```python
from build123d import *

# Parameters (mm, degrees)
SKETCH1_W               = 46.5
SKETCH1_H               = 24
BOSS_EXTRUDE1_DEPTH     = 21
SHELL1_T                = -1.25
SKETCH2_W               = 19.75
SKETCH2_H               = 14.5
CUT_EXTRUDE1_DEPTH      = 57.384838388
CUT_EXTRUDE4_REACH      = 57.358
SKETCH6_R               = 1.95
CUT_EXTRUDE5_REACH      = 57.358
SKETCH7_W               = 10.375
SKETCH7_H               = 2.5
SKETCH9_W               = 19.5
SKETCH9_H               = 6
BOSS_EXTRUDE3_DEPTH     = 2.5
CUT_EXTRUDE7_DEPTH      = 102.634838388
CUT_EXTRUDE7_DEPTH_BACK = 57.384838388
CUT_EXTRUDE7_START      = -45.25
SKETCH12_W              = 1.5
SKETCH12_H              = 8.25
SKETCH13_W              = 2.75
SKETCH13_H              = 8.25
BOSS_EXTRUDE4_DEPTH     = 44
SKETCH15_W              = 10
SKETCH15_H              = 2.75
BOSS_EXTRUDE5_DEPTH     = 0.75
CUT_EXTRUDE8_REACH      = 57.358
SKETCH18_W              = 6.76
SKETCH18_H              = 5
CUT_EXTRUDE9_REACH      = 57.358
SKETCH22_W              = 8.593751287
SKETCH22_H              = 16.011767213
CUT_EXTRUDE15_REACH     = 57.358
SKETCH25_W              = 10
SKETCH25_H              = 4.5


with BuildPart() as part:
    # Sketch1 → Boss-Extrude1 (new body)
    with BuildSketch(Plane.XY):
        with Locations((22, 12)):
            Rectangle(SKETCH1_W, SKETCH1_H)
    extrude(amount=-BOSS_EXTRUDE1_DEPTH)

    # Shell1
    shell1_openings = [part.faces().sort_by_distance(p)[0] for p in [
        (22, 12, -21),
        (22, 24, -10.5),
    ]]
    offset(amount=SHELL1_T, openings=shell1_openings, kind=Kind.INTERSECTION)

    # Sketch2 → Cut-Extrude1 (cut, through all)
    with BuildSketch(Plane.ZY.offset(1.25)):
        with Locations((-11.125, 8.5)):
            Rectangle(SKETCH2_W, SKETCH2_H)
    extrude(amount=-CUT_EXTRUDE1_DEPTH, mode=Mode.SUBTRACT)

    # Sketch6 → Cut-Extrude4 (cut, up to next)
    with BuildSketch(Plane(origin=(0, 0, 0), x_dir=(-1, 0, 0), z_dir=(0, -1, 0)), mode=Mode.PRIVATE) as cut_extrude4_sk1:
        with Locations(Location((-6.125, 9, 0), (0, 0, 90))):
            Circle(SKETCH6_R)
    cut_extrude4_tool1 = extrude(cut_extrude4_sk1.sketch, amount=-CUT_EXTRUDE4_REACH, mode=Mode.PRIVATE) & part.part
    # Sketch6 → Cut-Extrude4 (cut, up to next)
    with BuildSketch(Plane(origin=(0, 0, 0), x_dir=(-1, 0, 0), z_dir=(0, -1, 0)), mode=Mode.PRIVATE) as cut_extrude4_sk2:
        with Locations(Location((-37.875, 9, 0), (0, 0, 90))):
            Circle(SKETCH6_R)
    cut_extrude4_tool2 = extrude(cut_extrude4_sk2.sketch, amount=-CUT_EXTRUDE4_REACH, mode=Mode.PRIVATE) & part.part
    add(cut_extrude4_tool1.solids().sort_by_distance((6.125, 0, -9))[0], mode=Mode.SUBTRACT)
    add(cut_extrude4_tool2.solids().sort_by_distance((37.875, 0, -9))[0], mode=Mode.SUBTRACT)

    # Sketch7 → Cut-Extrude5 (cut, up to next)
    with BuildSketch(Plane.XY, mode=Mode.PRIVATE) as cut_extrude5_sk1:
        with Locations((40.0625, 2.5)):
            Rectangle(SKETCH7_W, SKETCH7_H)
    cut_extrude5_tool1 = extrude(cut_extrude5_sk1.sketch, amount=-CUT_EXTRUDE5_REACH, mode=Mode.PRIVATE) & part.part
    # Sketch7 → Cut-Extrude5 (cut, up to next)
    with BuildSketch(Plane.XY, mode=Mode.PRIVATE) as cut_extrude5_sk2:
        with Locations((3.9375, 2.5)):
            Rectangle(SKETCH7_W, SKETCH7_H)
    cut_extrude5_tool2 = extrude(cut_extrude5_sk2.sketch, amount=-CUT_EXTRUDE5_REACH, mode=Mode.PRIVATE) & part.part
    add(cut_extrude5_tool1.solids().sort_by_distance((40.0625, 2.5, 0))[0], mode=Mode.SUBTRACT)
    add(cut_extrude5_tool2.solids().sort_by_distance((3.9375, 2.5, 0))[0], mode=Mode.SUBTRACT)

    # Sketch9 → Boss-Extrude3 (add)
    with BuildSketch(Plane(origin=(0, 1.25, 0), x_dir=(1, 0, 0), z_dir=(0, 1, 0))):
        with Locations((25.125, 18)):
            Rectangle(SKETCH9_W, SKETCH9_H)
    extrude(amount=BOSS_EXTRUDE3_DEPTH)

    # Sketch12 → Cut-Extrude7 (cut, two sides: drawn at the far end of the back side and taken through both)
    with BuildSketch(Plane(origin=(45.25, 0, 0), x_dir=(0, 0, -1), z_dir=(1, 0, 0)).offset(CUT_EXTRUDE7_START - CUT_EXTRUDE7_DEPTH_BACK)):
        with Locations((20.25, 19.875)):
            Rectangle(SKETCH12_W, SKETCH12_H)
    extrude(amount=CUT_EXTRUDE7_DEPTH + CUT_EXTRUDE7_DEPTH_BACK, mode=Mode.SUBTRACT)

    # Sketch13 → Boss-Extrude4 (add)
    with BuildSketch(Plane(origin=(0, 0, 0), x_dir=(0, 0, -1), z_dir=(1, 0, 0))):
        with Locations((18.125, 19.875)):
            Rectangle(SKETCH13_W, SKETCH13_H)
    extrude(amount=BOSS_EXTRUDE4_DEPTH)

    # Sketch15 → Boss-Extrude5 (add)
    with BuildSketch(Plane.XZ.offset(-15.75)):
        with Locations((29.875, -18.125)):
            Rectangle(SKETCH15_W, SKETCH15_H)
    extrude(amount=BOSS_EXTRUDE5_DEPTH)

    # Sketch18 → Cut-Extrude8 (cut, up to next)
    with BuildSketch(Plane.XY, mode=Mode.PRIVATE) as cut_extrude8_sk1:
        with Locations((9.98, 10.1)):
            Rectangle(SKETCH18_W, SKETCH18_H)
    cut_extrude8_tool1 = extrude(cut_extrude8_sk1.sketch, amount=-CUT_EXTRUDE8_REACH, mode=Mode.PRIVATE) & part.part
    add(cut_extrude8_tool1.solids().sort_by_distance((9.98, 10.1, 0))[0], mode=Mode.SUBTRACT)

    # Sketch22 → Cut-Extrude9 (cut, up to next)
    with BuildSketch(Plane.XY, mode=Mode.PRIVATE) as cut_extrude9_sk1:
        with Locations((21.422492142, 15.994116394)):
            Rectangle(SKETCH22_W, SKETCH22_H)
    cut_extrude9_tool1 = extrude(cut_extrude9_sk1.sketch, amount=-CUT_EXTRUDE9_REACH, mode=Mode.PRIVATE) & part.part
    add(cut_extrude9_tool1.solids().sort_by_distance((21.422492, 15.994116, 0))[0], mode=Mode.SUBTRACT)

    # Sketch25 → Cut-Extrude15 (cut, up to next)
    with BuildSketch(Plane.XY, mode=Mode.PRIVATE) as cut_extrude15_sk1:
        Polygon((31.35, 18.75), (41.85, 18.75), (41.85, 24), (41.6, 24), (41.6, 19.5), (31.6, 19.5), (31.6, 24), (31.35, 24), align=None)
    cut_extrude15_tool1 = extrude(cut_extrude15_sk1.sketch, amount=-CUT_EXTRUDE15_REACH, mode=Mode.PRIVATE) & part.part
    # Sketch25 → Cut-Extrude15 (cut, up to next)
    with BuildSketch(Plane.XY, mode=Mode.PRIVATE) as cut_extrude15_sk2:
        with Locations((36.6, 21.75)):
            Rectangle(SKETCH25_W, SKETCH25_H)
    cut_extrude15_tool2 = extrude(cut_extrude15_sk2.sketch, amount=-CUT_EXTRUDE15_REACH, mode=Mode.PRIVATE) & part.part
    add(cut_extrude15_tool1.solids().sort_by_distance((31.475, 23.882606, 0))[0], mode=Mode.SUBTRACT)
    add(cut_extrude15_tool2.solids().sort_by_distance((36.6, 21.75, 0))[0], mode=Mode.SUBTRACT)


solid = part.part
```
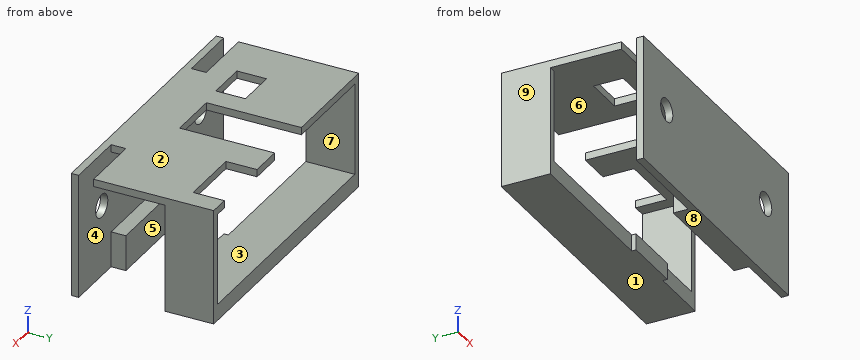
Geometry check sheet. Reference: the model listing, model coordinates, mm. Face numbers are marked on the shaded views. A direction names the side the tool comes from. Coordinates: 2 decimals unless noted, no trailing zeros. Loops run counter-clockwise (first coordinate to the right, second up) from the corner with the lowest first, then second, coordinate; pieces in that order, holes last. Notation, with made-up numbers: (-5.75, 11.25) - (37.25, 11.25) arc R28 ccw to (37.25, 30.25) - close; hole circle Ø6 at (59.25, 52.25). An arc over 180 degrees is marked (long way). One line per item, written item: value. Start each with the question number.
(1) Tool access check on the marked faces 1, 2, 3, 4 and 5. Record the directions out of +Z, -Z, +X, -X, +Y, -Y that give a thin tool (end or side, any length) a straight path to the whole face; none if there is none.
(2) Cross-section at B-B on y = 20. Enter the section's corners in (x, z).
(3) Mould release check, pull along Z, two halves, no side actions. Record for the marked faces 6, 7, 8 and 9: released by +Z, released by -Z, zero draft, split by the parting line, or undercut.
(4) Cross-section at A-A on z = -2.5. Enter the section's corners in (x, y), plus the area to 4 significant figures.
(5) Material ranges on line 1 (X direction, y = 0.9, z = -9) (3 decimals); line 2 (Y direction, x = 43.5, z = -17.25); line 3 (Y direction, x = 28, z = -19.25), recorded low to high. Write a range as [from, to].
(6) Cross-section at C-C on z = -9. Enter the section's corners in (x, y) (3 decimals).
(7) Cross-section at D-D on z = -17.5. Enter the section's corners in (x, y) (3 decimals), plus the area to 3 significant figures.
(8) Depth check by flat-ended pin: P1, Ø6, axis at x = 40.5, z = -16, coming from the -Y side; P2, Ø2, axis at x = 39.5, y = 12, coming from the -Z side; P3, Ø1.4, axis at y = 2.5, z = -0.5, coming from the -X side (3 decimals); P4, Ø2, axis at y = 14.5, z = -18, coming from the +X side (3 decimals). Enter the tip coordinate at first touch or a pass-through.
Results below:
1. face 1: -Z, +X, -X, +Y
1. face 2: +Z, +X, -X, +Y, -Y
1. face 3: +Y
1. face 4: none
1. face 5: -Z, +X, -X
2. outline: (-1.25, -19.5) - (45.25, -19.5) - (45.25, 0) - (41.85, 0) - (41.85, -1.25) - (44, -1.25) - (44, -16.75) - (0, -16.75) - (0, -1.25) - (17.13, -1.25) - (17.13, 0) - (-1.25, 0) - close; (25.72, -1.25) - (31.35, -1.25) - (31.35, 0) - (25.72, 0) - close
3. face 6: undercut
3. face 7: undercut
3. face 8: released by -Z
3. face 9: zero draft
4. outline: (-1.25, 0) - (45.25, 0) - (45.25, 1.25) - (-1.25, 1.25) - close; (-1.25, 15.75) - (0, 15.75) - (0, 24) - (-1.25, 24) - close; (44, 15.75) - (45.25, 15.75) - (45.25, 24) - (44, 24) - close
4. area: 78.75 mm2
5. line 1: x = [-1.25, 4.175], [8.075, 35.925], [39.825, 45.25]
5. line 2: y = [0, 1.25], [15.75, 24]
5. line 3: y = [0, 3.75], [15, 24]
6. outline: (-1.25, 0) - (4.175, 0) - (4.175, 1.25) - (-1.25, 1.25) - close; (-1.25, 15.75) - (0, 15.75) - (0, 24) - (-1.25, 24) - close; (8.075, 0) - (35.925, 0) - (35.925, 1.25) - (8.075, 1.25) - close; (39.825, 0) - (45.25, 0) - (45.25, 1.25) - (39.825, 1.25) - close; (44, 15.75) - (45.25, 15.75) - (45.25, 24) - (44, 24) - close
7. outline: (-1.25, 0) - (45.25, 0) - (45.25, 1.25) - (34.875, 1.25) - (34.875, 3.75) - (15.375, 3.75) - (15.375, 1.25) - (-1.25, 1.25) - close; (-1.25, 15.75) - (24.875, 15.75) - (24.875, 15) - (34.875, 15) - (34.875, 15.75) - (45.25, 15.75) - (45.25, 24) - (-1.25, 24) - close
7. area: 498 mm2
8. P1: stops at y = 0
8. P2: stops at z = -1.25
8. P3: stops at x = 9.125
8. P4: stops at x = 34.875
